Autodesk Inventor part; units mm, degrees
ref_plane "YZ Plane" through (0, 0, 0) normal (1, 0, 0) x (0, 1, 0)
ref_plane "XZ Plane" through (0, 0, 0) normal (0, 1, 0) x (-1, 0, 0)
ref_plane "XY Plane" through (0, 0, 0) normal (0, 0, 1) x (1, 0, 0)
sketch "スケッチ1" plane through (0, 0, 0) normal (0, 1, 0) x (-1, 0, 0)
  line L0 (-9, 20) -> (9, 20)
  line L1 (12, 17) -> (12, -17)
  line L2 (9, -20) -> (-9, -20)
  line L3 (-12, -17) -> (-12, 17)
  line L4 (-12, 20) -> (12, -20) construction
  line L5 (12, 20) -> (-12, -20) construction
  line L6 (0, -28.8698) -> (0, 28.8698)
  circle A0 centre (8, 8.2) radius 2.425
  circle A1 centre (-8, 8.2) radius 2.425
  arc A2 (12, 17) -> (9, 20) centre (9, 17) ccw
  arc A3 (-9, 20) -> (-12, 17) centre (-9, 17) ccw
  arc A4 (-12, -17) -> (-9, -20) centre (-9, -17) ccw
  arc A5 (9, -20) -> (12, -17) centre (9, -17) ccw
  point P0 (0, 0)
  dimension "d0" = 24
  dimension "d1" = 40
  dimension "d4" = 4.85
  dimension "d5" = 16
  dimension "d6" = 11.8
  dimension "d7" = 3
extrude "押し出し1" add sketch "スケッチ1" along normal blind 8.3
sketch "スケッチ2" plane through (0, 8.3, 0) normal (0, 1, 0) x (1, 0, 0)
  line L0 (-12, 17) -> (-12, -17)
  line L1 (-9, 2.5) -> (9, 2.5)
  line L2 (12, -17) -> (12, 17)
  line L3 (-12, 17) -> (-12, 5.5)
  line L4 (12, 17) -> (12, 5.5)
  arc A0 (-12, 5.5) -> (-9, 2.5) centre (-9, 5.5) ccw
  arc A1 (9, 2.5) -> (12, 5.5) centre (9, 5.5) ccw
  line L5 (9, 20) -> (-9, 20)
  arc A2 (-9, 20) -> (-12, 17) centre (-9, 17) ccw
  arc A3 (12, 17) -> (9, 20) centre (9, 17) ccw
  point P0 (0, 0)
  point P1 (-12, 2.5)
  point P2 (12, 2.5)
  dimension "d10" = 3
  dimension "d11" = 17.5
extrude "押し出し2" add sketch "スケッチ2" along normal blind 4.4
sketch "スケッチ3" plane through (0, 12.7, 0) normal (0, 1, 0) x (1, 0, 0)
  circle A0 centre (0, 11.25) radius 7
  line L0 (-12, 17) -> (-12, 5.5)
  line L1 (-12, 11.25) -> (12, 11.25) construction
  line L2 (12, 5.5) -> (12, 17)
  line L3 (9, 20) -> (-9, 20)
  line L4 (0, 20) -> (0, 2.5) construction
  line L5 (-9, 2.5) -> (9, 2.5)
  point P0 (0, 0)
  dimension "d14" = 14
extrude "押し出し3" add sketch "スケッチ3" along normal blind 3
fillet "フィレット1" radius 0.5 1 edges at (-7, 15.7, -11.25)
fillet "フィレット2" radius 0.5 21 edges at (11.1213, 8.3, 19.1213) (0, 8.3, 20) (-11.1213, 8.3, 19.1213) (-12, 8.3, 5.75) (12, 8.3, 5.75) (11.1213, 12.7, -3.3787) (12, 12.7, -11.25) (11.1213, 12.7, -19.1213) (0, 12.7, -20) (-11.1213, 12.7, -19.1213) (-12, 12.7, -11.25) (-11.1213, 12.7, -3.3787) (0, 12.7, -2.5) (11.1213, 0, 19.1213) (12, 0, 0) (11.1213, 0, -19.1213) (0, 0, -20) (-11.1213, 0, -19.1213) (-12, 0, 0) (-11.1213, 0, 19.1213) (0, 0, 20)
sketch "スケッチ4" plane through (0, 0, 0) normal (1, 0, 0) x (0, 1, 0)
  line L0 (10.3657, 22.992) -> (3.1274, 22.992)
  line L1 (3.1274, 22.992) -> (3.1274, 14.1637)
  line L2 (3.1274, 14.1637) -> (10.3657, 14.1637)
  line L3 (10.3657, 14.1637) -> (10.3657, 22.992)
  point P0 (0, 0)
extrude "押し出し4" cut sketch "スケッチ4" along normal mid plane 8
fillet "フィレット3" radius 0.5 12 edges at (0, 8.3, 14.1637) (-4, 8.1536, 19.8536) (-4, 5.4637, 20) (-4, 8.3, 16.8319) (-4, 5.7137, 14.1637) (-4, 3.1274, 17.0819) (0, 3.1274, 14.1637) (4, 8.1536, 19.8536) (4, 8.3, 16.8319) (4, 5.4637, 20) (0, 3.1274, 20) (4, 5.7137, 14.1637)
properties part number "UnitV_OV7740_M12"
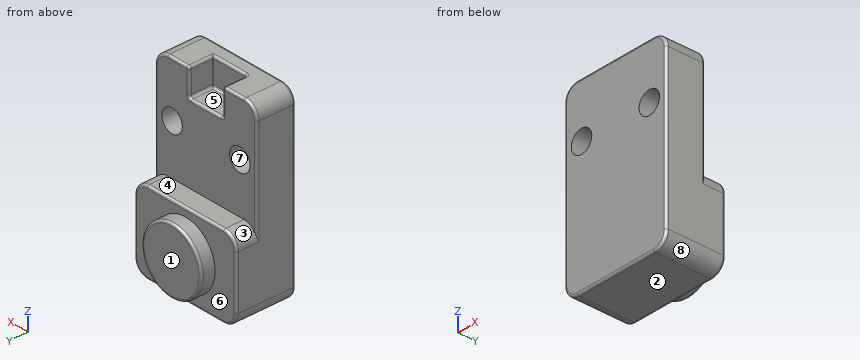
Model file for the job. Use its own axes, mm. Face numbers are marked on the shaded views. A direction names the side the tool comes from. Give positions to 0.01 mm unless a question says otherwise; leave off trailing zeros. Loops run counter-clockwise (first coordinate to the right, second up) from the corner with the lowest first, then second, coordinate; pieces in that order, holes last. Notation, with made-up numbers: (-19.5, -36) - (-8.5, -36) arc R19 ccw to (-8.5, -26) - close; hole circle Ø8 at (54, 47). An arc over 180 degrees is marked (long way). One line per item, written item: value. Start each with the question number.
1. Slice it at B-B (y = 1). List the corners of the cut face in (x, z) (3 decimals).
2. Slice it at A-A (x = -8). List the corners of the cut face in (y, z) (3 decimals).
3. Which spindle directions (+Z, -Z, +X, -X, +Y, -Y) get a long thin tool onto all of the face, cutting with end or side? Do the marked faces 1, 2, 3, 4 and 5. Say none if no direction does.
4. Probe L1, parallel to Z at x = -8, y = 4.5 (3 decimals); L2, parallel to Z at x = 1.5, y = 9.5; L3, parallel to X at y = 3, z = 7.5. List the from-to ranges inside material, lowest first. Write a range as from..to.
5. Slice it at D-D (z = 10). List the corners of the cut face in (x, y) (3 decimals).
6. Pin check, flat tips, straight feed: pin 1 (1.3 mm diameter, centred on x = -1, y = 5.5, fed in from +Z); pin 2 (5.5 mm diameter, centred on x = 1, z = 18, fed in from +Y); pin 3 (8 mm diameter, centred on x = 8, z = 8.2, fed in from +Y). Stop position of each tip, or through.
7. Pull direction X, two halves, no side cores. Call the marked faces 6, 7 and 8: pulls with the +X half, pulls with the -X half, needs draft (parallel to the pull), parting line crosses it, or undercut.
8. Slice it at C-C (z = -11.25). List the corners of the cut face in (x, y), plus the area to 3 significant figures.
Solution:
1. outline: (-12, -17) arc R3 ccw to (-9, -20) - (9, -20) arc R3 ccw to (12, -17) - (12, 17) arc R3 ccw to (9, 20) - (-9, 20) arc R3 ccw to (-12, 17) - close; hole circle Ø4.85 at (-8, 8.2); hole circle Ø4.85 at (8, 8.2)
2. outline: (0, -19.5) arc R0.5 ccw to (0.5, -20) - (12.2, -20) arc R0.5 ccw to (12.7, -19.5) - (12.7, -3) arc R0.5 ccw to (12.2, -2.5) - (8.3, -2.5) - (8.3, 5.775) - (0, 5.775) - close; (0, 10.625) - (8.3, 10.625) - (8.3, 19.5) arc R0.5 ccw to (7.8, 20) - (0.5, 20) arc R0.5 ccw to (0, 19.5) - close
3. face 1: +Z, -Z, +X, -X, +Y
3. face 2: -Z, +X, -X, +Y, -Y
3. face 3: +Z, -X, +Y
3. face 4: +Z, +X, -X, +Y
3. face 5: +Z, +Y
4. L1: z = -20..5.775, 10.625..20
4. L2: z = -20..-2.5
4. L3: x = -12..-10.32, -5.68..5.68, 10.32..12
5. outline: (-12, 0.5) arc R0.5 ccw to (-11.5, 0) - (-9.625, 0) - (-9.625, 8.3) - (-11.5, 8.3) arc R0.5 ccw to (-12, 7.8) - close; (-6.375, 0) - (6.375, 0) - (6.375, 8.3) - (-6.375, 8.3) - close; (9.625, 0) - (11.5, 0) arc R0.5 ccw to (12, 0.5) - (12, 7.8) arc R0.5 ccw to (11.5, 8.3) - (9.625, 8.3) - close
6. pin 1: stops at z = 14.16
6. pin 2: stops at y = 3.13
6. pin 3: stops at y = 8.3
7. face 6: needs draft
7. face 7: undercut
7. face 8: pulls with the +X half
8. outline: (-12, 0.5) arc R0.5 ccw to (-11.5, 0) - (11.5, 0) arc R0.5 ccw to (12, 0.5) - (12, 12.2) arc R0.5 ccw to (11.5, 12.7) - (7, 12.7) - (7, 15.2) arc R0.5 ccw to (6.5, 15.7) - (-6.5, 15.7) arc R0.5 ccw to (-7, 15.2) - (-7, 12.7) - (-11.5, 12.7) arc R0.5 ccw to (-12, 12.2) - close
8. area: 346 mm^2
